from build123d import *

# Parameters (mm, degrees)
EXTRUDE_1_DEPTH     = 3
CUT_EXTRUDE_1_REACH = 52.09
SKETCH_2_R          = 1.6
FILLET_1_R          = 3
FILLET_2_R          = 3


with BuildPart() as part:
    # 草图1 → 凸台-拉伸1 (new body)
    with BuildSketch(Plane.XY):
        Polygon((-20, 20), (-30, 20), (-30, 40), (30, 40), (30, 20), (20, 20), (20, -20), (-20, -20), align=None)
    extrude(amount=EXTRUDE_1_DEPTH)

    # 草图2 → 切除-拉伸1 (cut, up to next)
    with BuildSketch(Plane.XY.offset(3), mode=Mode.PRIVATE) as cut_extrude_1_sk1:
        with Locations((-20, 30)):
            Circle(SKETCH_2_R)
    cut_extrude_1_tool1 = extrude(cut_extrude_1_sk1.sketch, amount=-CUT_EXTRUDE_1_REACH, mode=Mode.PRIVATE) & part.part
    # 草图2 → 切除-拉伸1 (cut, up to next)
    with BuildSketch(Plane.XY.offset(3), mode=Mode.PRIVATE) as cut_extrude_1_sk2:
        with Locations((0, 30)):
            Circle(SKETCH_2_R)
    cut_extrude_1_tool2 = extrude(cut_extrude_1_sk2.sketch, amount=-CUT_EXTRUDE_1_REACH, mode=Mode.PRIVATE) & part.part
    # 草图2 → 切除-拉伸1 (cut, up to next)
    with BuildSketch(Plane.XY.offset(3), mode=Mode.PRIVATE) as cut_extrude_1_sk3:
        with Locations((20, 30)):
            Circle(SKETCH_2_R)
    cut_extrude_1_tool3 = extrude(cut_extrude_1_sk3.sketch, amount=-CUT_EXTRUDE_1_REACH, mode=Mode.PRIVATE) & part.part
    # 草图2 → 切除-拉伸1 (cut, up to next)
    with BuildSketch(Plane.XY.offset(3), mode=Mode.PRIVATE) as cut_extrude_1_sk4:
        with Locations((-10, -10)):
            Circle(SKETCH_2_R)
    cut_extrude_1_tool4 = extrude(cut_extrude_1_sk4.sketch, amount=-CUT_EXTRUDE_1_REACH, mode=Mode.PRIVATE) & part.part
    # 草图2 → 切除-拉伸1 (cut, up to next)
    with BuildSketch(Plane.XY.offset(3), mode=Mode.PRIVATE) as cut_extrude_1_sk5:
        with Locations((10, -10)):
            Circle(SKETCH_2_R)
    cut_extrude_1_tool5 = extrude(cut_extrude_1_sk5.sketch, amount=-CUT_EXTRUDE_1_REACH, mode=Mode.PRIVATE) & part.part
    # 草图2 → 切除-拉伸1 (cut, up to next)
    with BuildSketch(Plane.XY.offset(3), mode=Mode.PRIVATE) as cut_extrude_1_sk6:
        with Locations((10, 10)):
            Circle(SKETCH_2_R)
    cut_extrude_1_tool6 = extrude(cut_extrude_1_sk6.sketch, amount=-CUT_EXTRUDE_1_REACH, mode=Mode.PRIVATE) & part.part
    # 草图2 → 切除-拉伸1 (cut, up to next)
    with BuildSketch(Plane.XY.offset(3), mode=Mode.PRIVATE) as cut_extrude_1_sk7:
        with Locations((-10, 10)):
            Circle(SKETCH_2_R)
    cut_extrude_1_tool7 = extrude(cut_extrude_1_sk7.sketch, amount=-CUT_EXTRUDE_1_REACH, mode=Mode.PRIVATE) & part.part
    add(cut_extrude_1_tool1.solids().sort_by_distance((-20, 30, 3))[0], mode=Mode.SUBTRACT)
    add(cut_extrude_1_tool2.solids().sort_by_distance((0, 30, 3))[0], mode=Mode.SUBTRACT)
    add(cut_extrude_1_tool3.solids().sort_by_distance((20, 30, 3))[0], mode=Mode.SUBTRACT)
    add(cut_extrude_1_tool4.solids().sort_by_distance((-10, -10, 3))[0], mode=Mode.SUBTRACT)
    add(cut_extrude_1_tool5.solids().sort_by_distance((10, -10, 3))[0], mode=Mode.SUBTRACT)
    add(cut_extrude_1_tool6.solids().sort_by_distance((10, 10, 3))[0], mode=Mode.SUBTRACT)
    add(cut_extrude_1_tool7.solids().sort_by_distance((-10, 10, 3))[0], mode=Mode.SUBTRACT)

    # 圆角1
    fillet_1_edges = [part.edges().sort_by_distance(p)[0] for p in [
        (20, -20, 1.5),
        (-20, -20, 1.5),
        (-30, 20, 1.5),
        (-30, 40, 1.5),
        (30, 40, 1.5),
        (30, 20, 1.5),
    ]]
    fillet(fillet_1_edges, radius=FILLET_1_R)

    # 圆角2
    fillet_2_edges = [part.edges().sort_by_distance(p)[0] for p in [
        (-20, 20, 1.5),
        (20, 20, 1.5),
    ]]
    fillet(fillet_2_edges, radius=FILLET_2_R)


solid = part.part
Part model, mm, in its own coordinate system. A direction names the side the tool comes from. Coordinates: 2 decimals unless noted, no trailing zeros. Order: outer loops, then holes, each group sorted by start corner. A loop starts at its lowest first (then second) coordinate and runs counter-clockwise, first axis right, second up. Notation, with made-up numbers: M 57,17.5 L 91,17.5 A21 cw 91,38.5 Z; hole C -36.75,82.25 d8. An arc over 180 degrees is marked long. Use a Markdown table: item, result.
(1) Cut at C-C on x = 0. Write the cut outline in (y, z).
A:
| item | result |
|---|---|
| outline | M -20,0 L 28.4,0 L 28.4,3 L -20,3 Z; M 31.6,0 L 40,0 L 40,3 L 31.6,3 Z |
(2) Cut at D-D on z = 0.6. Write the cut outline in (x, y), then the cut area to 3 significant figures.
A:
| item | result |
|---|---|
| outline | M -30,23 A3 ccw -27,20 L -23,20 A3 cw -20,17 L -20,-17 A3 ccw -17,-20 L 17,-20 A3 ccw 20,-17 L 20,17 A3 cw 23,20 L 27,20 A3 ccw 30,23 L 30,37 A3 ccw 27,40 L -27,40 A3 ccw -30,37 Z; hole C -20,30 d3.2; hole C -10,-10 d3.2; hole C -10,10 d3.2; hole C 0,30 d3.2; hole C 10,-10 d3.2; hole C 10,10 d3.2; hole C 20,30 d3.2 |
| area | 2,740 mm^2 |
(3) Cut at A-A on x = 10. Write the cut outline in (y, z), then the cut area to 3 significant figures.
A:
| item | result |
|---|---|
| outline | M -20,0 L -11.6,0 L -11.6,3 L -20,3 Z; M -8.4,0 L 8.4,0 L 8.4,3 L -8.4,3 Z; M 11.6,0 L 40,0 L 40,3 L 11.6,3 Z |
| area | 161 mm^2 |
(4) Tool access for faces 1 (the flat face through (-20, 0, 1)), 2 (the flat face through (20, 0, 1)), 3 (the cylindrical face through (-20.208, 31.586, 1.521)): list every direction of +Z, -Z, +X, -X, +Y, -Y with a clear straight run to the whole face (end or side of a thin tool).
A:
| item | result |
|---|---|
| face 1 | +Z, -Z, -X, -Y |
| face 2 | +Z, -Z, +X, -Y |
| face 3 | +Z, -Z |
(5) Flat gauge pins, fed straight in: pin 1 (0.9 mm diameter, centred on x = -25.5, z = 1, fed in from -Y); pin 2 (0.9 mm diameter, centred on y = -6, z = 1, fed in from -X); pin 3 (1.5 mm diameter, centred on y = -8, z = 1.5, fed in from +X); pin 4 (2.5 mm diameter, centred on x = -20, y = 30, fed in from -Z). Where does each tip first touch, or does it go through?
A:
| item | result |
|---|---|
| pin 1 | stops at y = 20 |
| pin 2 | stops at x = -20 |
| pin 3 | stops at x = 20 |
| pin 4 | passes through |
(6) Pull direction X, two halves, no side cores. Call faces 4 (the cylindrical face through (-29.1, 20.86, 1.52)), 5 (the cylindrical face through (18.82, 31.08, 1.52)), 6 (the cylindrical face through (19.1, -19.14, 1.52)): released by +X, released by -X, zero draft, split by the parting line, or undercut.
A:
| item | result |
|---|---|
| face 4 | released by -X |
| face 5 | undercut |
| face 6 | released by +X |
(7) Probe L1, parallel to Y at x = 0, z = 1.3; L2, parallel to X at y = 2, z = 0.2; L3, parallel to Y at x = -26, z = 1.25. List the from-to ranges inside material, lowest first.
A:
| item | result |
|---|---|
| L1 | y = -20 to 28.4, 31.6 to 40 |
| L2 | x = -20 to 20 |
| L3 | y = 20 to 40 |
(8) Cut at B-B on y = -10. Write the cut outline in (x, z), then the cut area to 3 significant figures.
A:
| item | result |
|---|---|
| outline | M -20,0 L -11.6,0 L -11.6,3 L -20,3 Z; M -8.4,0 L 8.4,0 L 8.4,3 L -8.4,3 Z; M 11.6,0 L 20,0 L 20,3 L 11.6,3 Z |
| area | 101 mm^2 |
